```python
from build123d import *

# Parameters (mm, degrees)
PAD_DEPTH    = 1.6
SKETCH_R     = 2
PAD001_DEPTH = 20


with BuildPart() as part:
    # Sketch001 → Pad (new body, symmetric)
    with BuildSketch(Plane(origin=(0, 0, 0), x_dir=(1, 0, 0), z_dir=(0, 0, -1))):
        Polygon((4.041452, 0), (2.020726, 3.5), (-2.020726, 3.5), (-4.041452, 0), (-2.020726, -3.5), (2.020726, -3.5), align=None)
    extrude(amount=PAD_DEPTH, both=True)

    # Sketch (on Face7 of Pad) → Pad001 (join)
    with BuildSketch(Plane.XY.offset(1.6)):
        Circle(SKETCH_R)
    extrude(amount=PAD001_DEPTH)

    # Sketch002 → Groove (revolve, cut)
    with BuildSketch(Plane.XZ):
        Polygon((3.100253, 2.054888), (4.213852, 0.941288), (4.213852, -0.941288), (3.100253, -2.054888), (5.186611, -2.054888), (5.186611, 2.054888), align=None)
    revolve(axis=Axis((0, 0, 0), (0, 0, 1)), mode=Mode.SUBTRACT)


solid = part.part
```
Work out the finished part from the listing and answer in its coordinate system (mm). A direction names the side the tool comes from. Give positions to 0.01 mm unless a question says otherwise; leave off trailing zeros. Loops run counter-clockwise (first coordinate to the right, second up) from the corner with the lowest first, then second, coordinate; pieces in that order, holes last. Notation, with made-up numbers: M -5,32.5 L -1,32.5 A33 ccw -1,70.5 Z; hole C 83,27 d9. An arc over 180 degrees is marked long. One line per item, written item: value. Start each with the question number.
1. Which of the six approach directions +Z, -Z, +X, -X, +Y, -Y give full straight-line access (tool end or side, diameter ignored) to faces 1 (the face through (-1.86, -3.19, 1.46)), 2 (the face through (0, -2, 11))?
2. Find section B-B (z = 3.5). Give the vertices of the cut face in (x, y), and give its area (3 significant figures).
3. Find the intervals of material crossed by probe 1 along Z at (x, y) = (0, -2.25); probe 2 along X at (y, z) = (1.25, 5); probe 3 along Y at (x, z) = (0, 2), in increasing order.
4. Each of these flat-tipped pins is pushed along its axis until it touches: P1, Ø2, axis at x = 1, z = 9.5, coming from the +Y side; P2, Ø2, axis at y = -1, z = 15, coming from the -X side; P3, Ø4, axis at y = -1.5, z = 7, coming from the +X side. Where does it stop, or does it pass through?
5. Find section A-A (x = 0). Give the vertices of the cut face in (y, z), and give its area (3 significant figures).
Reported:
1. face 1: +Z, -X, -Y
1. face 2: +Z
2. outline: C 0,0 d4
2. area: 12.6 mm²
3. probe 1: z = -1.6 to 1.6
3. probe 2: x = -1.56 to 1.56
3. probe 3: y = -2 to 2
4. P1: stops at y = 2
4. P2: stops at x = -2
4. P3: stops at x = 2
5. outline: M -3.5,-1.6 L 3.5,-1.6 L 3.5,1.6 L 2,1.6 L 2,21.6 L -2,21.6 L -2,1.6 L -3.5,1.6 Z
5. area: 102 mm²
